from build123d import *

# Parameters (mm, degrees)
BOSS_EXTRUDE1_DEPTH = 6.35
SKETCH2_R           = 10.16
BOSS_EXTRUDE2_DEPTH = 6.35
FILLET1_R           = 10.16


with BuildPart() as part:
    # Sketch1 → Boss-Extrude1 (new body)
    with BuildSketch(Plane(origin=(0, 0, 0), x_dir=(1, 0, 0), z_dir=(0, 1, 0))):
        Polygon((40.933013594, 72.038381655), (-82.853575358, -0.570161201), (41.920561763, -71.468220453), align=None)
    extrude(amount=BOSS_EXTRUDE1_DEPTH)

    # Sketch2 → Boss-Extrude2 (add)
    with BuildSketch(Plane(origin=(0, 6.35, 0), x_dir=(1, 0, 0), z_dir=(0, 1, 0))):
        with Locations(Location((-62.534056475, -0.430331372, 0), (0, 0, 120.394277672))):
            Circle(SKETCH2_R)
        with Locations(Location((30.894350337, 54.371247195, 0), (0, 0, 120.394277672))):
            Circle(SKETCH2_R)
        with Locations(Location((31.639706138, -53.940915823, 0), (0, 0, 0.394277672))):
            Circle(SKETCH2_R)
    extrude(amount=BOSS_EXTRUDE2_DEPTH)

    # Fillet1
    fillet1_edges = [part.edges().sort_by_distance(p)[0] for p in [
        (40.933013594, 3.175, -72.038381655),
        (41.920561763, 3.175, 71.468220453),
        (-82.853575358, 3.175, 0.570161201),
    ]]
    fillet(fillet1_edges, radius=FILLET1_R - 0.0001)  # a hair under: the kernel refuses the full size


solid = part.part
The listing builds one solid part. Answer for the finished solid, in the listing's coordinates (mm). A direction names the side the tool comes from. Round coordinates to 2 decimals unless told otherwise and drop trailing zeros. Order: outer loops, then holes, each group sorted by start corner. A loop starts at its lowest first (then second) coordinate and runs counter-clockwise, first axis right, second up. Notation, with made-up numbers: (-37.75, 87) -> (17.25, 87) arc R13 ccw to (17.25, 103) -> close; hole circle Ø2 at (-26.75, -10). An arc over 180 degrees is marked (long way). One line per item, written item: value.
Item 1: Given P1, Ø5, axis at x = 13, y = 5, coming from the +Z side; P2, Ø5, axis at y = 5, z = 40.5, coming from the +X side; P3, Ø2, axis at x = 2, z = 22.5, coming from the +Y side, each flat-ended and moving along its own axis, determine where each tip first touches the part or whether it passes through.
Taken from the geometry:
P1: stops at z = 56.46
P2: stops at x = 41.72
P3: stops at y = 6.35
Item 2: For faces 4 (the cylindrical face through (36.297, 9.481, -62.976)), 5 (the flat face through (-4, 0, -1)), determine the directions among +Z, -Z, +X, -X, +Y, -Y from which every point of the face is accessible in a straight line to the end or side of a thin tool.
Taken from the geometry:
face 4: +Y
face 5: +Z, -Z, +X, -X, -Y
Item 3: Find section D-D, the plane x = -60. Give the vertices of the cut face in (y, z), then the cut area to 3 significant figures.
Taken from the geometry:
outline: (0, -12.83) -> (6.35, -12.83) -> (6.35, -9.41) -> (12.7, -9.41) -> (12.7, 10.27) -> (6.35, 10.27) -> (6.35, 13.56) -> (0, 13.56) -> close
area: 293 mm2
Item 4: Find section A-A, the plane y = 2.75. Give the vertices of the cut face in (x, z).
Taken from the geometry:
outline: (-67.67, -8.33) -> (25.75, -63.13) arc R10.16 ccw to (41.05, -54.44) -> (41.8, 53.87) arc R10.16 ccw to (26.62, 62.77) -> (-67.55, 9.26) arc R10.16 ccw to start
Item 5: For a pull along Z with two mould halves and no side action, classify faces 1 (the cylindrical face through (30.248, 9.481, 43.877)), 2 (the flat face through (31, 12.7, -54)), 3 (the cylindrical face through (-70.55, 9.48, 6.67)) as released by +Z, released by -Z, zero draft, split by the parting line, or undercut.
Taken from the geometry:
face 1: undercut
face 2: zero draft
face 3: split by the parting line
Item 6: Find section B-B, the plane z = 45.5. Give the vertices of the cut face in (x, y), then the cut area to 3 significant figures.
Taken from the geometry:
outline: (-3.78, 0) -> (41.74, 0) -> (41.74, 6.35) -> (37.29, 6.35) -> (37.29, 12.7) -> (25.98, 12.7) -> (25.98, 6.35) -> (-3.78, 6.35) -> close
area: 361 mm2
Item 7: Find section C-C, the plane y = 10. Give the vertices of the cut face in (x, z).
Taken from the geometry:
outline: circle Ø20.32 at (-62.53, 0.43); circle Ø20.32 at (30.89, -54.37); circle Ø20.32 at (31.64, 53.94)
Item 8: Straight lines are drawn through the part: L1, parallel to Y at x = 32, z = -7; L2, parallel to Z at x = -51, y = 2; L3, parallel to X at y = 0.75, z = -1. For each, find the intervals that lie inside material, in ascending order.
Taken from the geometry:
L1: y = 0 to 6.35
L2: z = -18.11 to 18.67
L3: x = -72.59 to 41.42
